from build123d import *

# Parameters (mm, degrees)
CROQUIS1_W              = 200
CROQUIS1_H              = 100
SALIENTE_EXTRUIR1_DEPTH = 10
CROQUIS2_W              = 180
CROQUIS2_H              = 80
CROQUIS3_W              = 180
CROQUIS3_H              = 80
CROQUIS4_R              = 7.5
CROQUIS4_R_2            = 15
CROQUIS4_R_3            = 22.5
CORTAR_EXTRUIR1_DEPTH   = 30
CHAFL_N2_SIZE           = 5


with BuildPart() as part:
    # Croquis1 → Saliente-Extruir1 (new body)
    with BuildSketch(Plane(origin=(0, 0, 0), x_dir=(1, 0, 0), z_dir=(0, 1, 0))):
        Rectangle(CROQUIS1_W, CROQUIS1_H)
    extrude(amount=SALIENTE_EXTRUIR1_DEPTH)

    # Croquis2 → section 0 of recubrir1
    with BuildSketch(Plane(origin=(0, -10, 0), x_dir=(1, 0, 0), z_dir=(0, 1, 0)), mode=Mode.PRIVATE) as recubrir1_s0:
        Rectangle(CROQUIS2_W, CROQUIS2_H)
    # loft up to a face of the part (recubrir1)
    loft([recubrir1_s0.sketch, part.faces().sort_by_distance((0, 0, 0))[0]])

    # Croquis3 → section 0 of recubrir2
    with BuildSketch(Plane(origin=(0, 20, 0), x_dir=(1, 0, 0), z_dir=(0, 1, 0)), mode=Mode.PRIVATE) as recubrir2_s0:
        Rectangle(CROQUIS3_W, CROQUIS3_H)
    # loft up to a face of the part (recubrir2)
    loft([recubrir2_s0.sketch, part.faces().sort_by_distance((0, 10, 0))[0]])

    # Croquis4 → Cortar-Extruir1 (cut)
    with BuildSketch(Plane(origin=(0, 20, 0), x_dir=(1, 0, 0), z_dir=(0, 1, 0))):
        with Locations((-75, 0)):
            Circle(CROQUIS4_R)
        with Locations((-25, 0)):
            Circle(CROQUIS4_R_2)
        with Locations((50, 0)):
            Circle(CROQUIS4_R_3)
    extrude(amount=-CORTAR_EXTRUIR1_DEPTH, mode=Mode.SUBTRACT)

    # Chaflán2
    chafl_n2_edges = [part.edges().sort_by_distance(p)[0] for p in [
        (-82.5, -10, 0),
        (-40, -10, 0),
        (27.5, -10, 0),
    ]]
    chamfer(chafl_n2_edges, length=CHAFL_N2_SIZE)


solid = part.part
Design review of the part built by this model. Coordinates are the model's own, in mm. Coordinates: 2 decimals unless noted, no trailing zeros. Write each loop counter-clockwise with the first axis right and the second up, starting at its lowest first coordinate (ties: lowest second). Pieces come first, ordered by that corner, then holes. Notation, with made-up numbers: (87.5, -37) - (105.5, -37) arc R34 cw to (105.5, -7) - close; hole circle Ø3 at (2, 59). An arc over 180 degrees is marked (long way). Use one line per item in the form item = value.
Q1. For probe 1 along X at (y, z) = (3.75, 0); probe 2 along X at (y, z) = (-4.5, 8.5); probe 3 along X at (y, z) = (14, 0), list the stretches that pass through material, from the lowest coordinate up.
Taken from the geometry:
probe_1 = -100 to -82.5, -67.5 to -40, -10 to 27.5, 72.5 to 100
probe_2 = -95.5 to -37.36, -12.64 to 29.17, 70.83 to 95.5
probe_3 = -96 to -82.5, -67.5 to -40, -10 to 27.5, 72.5 to 96
Q2. Insertion check: pin 1 Ø2 at (y, z) = (-3, -36.5) entering from -X. The pin has a flat end and moves straight along its axis. Give the tip position at first contact, or say it passes through.
Taken from the geometry:
pin_1 = -98
Q3. Consider section B-B (z = 0). Count the separate pieces of the cut face and the enclosed holes in it, plus the area to 4 significant figures.
Taken from the geometry:
separate_pieces = 4
enclosed_holes = 0
area = 3,025 mm^2
Q4. Consider section A-A (y = 6). Write out the cut boundary in (x, z), plus the area to 3 significant figures.
Taken from the geometry:
outline = (-100, -50) - (100, -50) - (100, 50) - (-100, 50) - close; hole circle Ø15 at (-75, 0); hole circle Ø30 at (-25, 0); hole circle Ø45 at (50, 0)
area = 17,500 mm^2
Q5. The part is to be moulded in two halves that separate along Z. For faces 1 (the flat face through (-1, 5, -50)), 2 (the conical face through (-10.855, -5.313, 5.865)), 3 (the flat face through (100, 5, 1)), say which applies: +Z half, -Z half, draft (parallel to the pull), parting line (faces both ways), or undercut.
Taken from the geometry:
face_1 = -Z half
face_2 = undercut
face_3 = draft
